Job drawing, mm, ordinate dimensions from the low corner. One solid piece. A direction names the side the tool comes from. Coordinates: 2 decimals unless noted, no trailing zeros. Loops run counter-clockwise (first coordinate to the right, second up) from the corner with the lowest first, then second, coordinate; pieces in that order, holes last. Notation, with made-up numbers: (57, 5.25) -> (63, 5.25) arc R26 cw to (63, 19.25) -> close; hole circle Ø5 at (75.5, 17.5). An arc over 180 degrees is marked (long way). Answer as CSV lines item,"result". Start each with the question number.
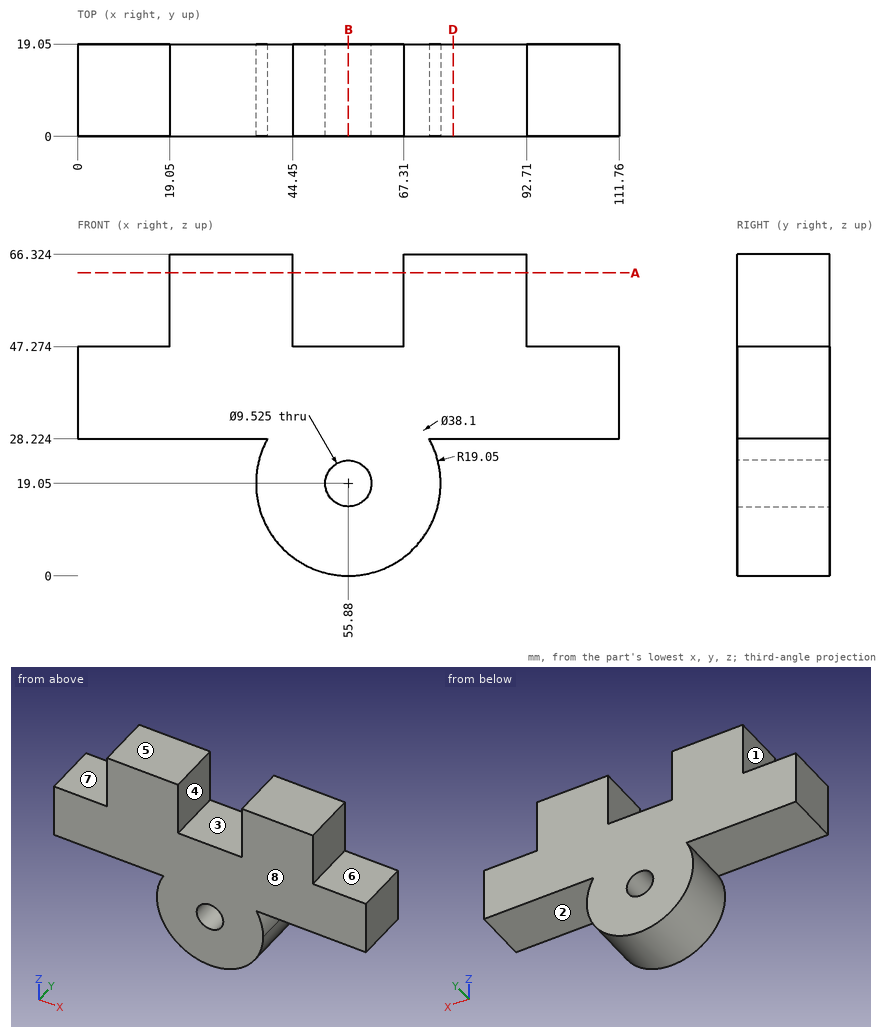
Q1. Two-plate mould, pull along X, no slides. Class the marked faces 1, 2 and 3: pulls with the +X half, pulls with the -X half, needs draft (parallel to the pull), parting line crosses it, or undercut.
Q2. Probe probe 1 along Z at (x, y) = (55.88, 5.5); probe 2 along Z at (x, y) = (95, 5.5); probe 3 along Z at (x, y) = (24.5, 14). List the from-to ranges inside material, lowest first. Write a range as from..to.
Q3. Which spindle directions (+Z, -Z, +X, -X, +Y, -Y) get a long thin tool onto all of the face, cutting with end or side? Do the marked faces 4, 5, 6, 7 and 8. Say none if no direction does.
Q4. Saw through at A-A (z = 62.5). List the corners of the cut face in (x, y), and give its area (3 significant figures).
Q5. Saw through at B-B (x = 55.88). List the corners of the cut face in (y, z).
Q6. Saw through at D-D (x = 77.5). List the corners of the cut face in (y, z).
Q7. Pin check, flat tips, straight feed: pin 1 Ø5.5 at (x, y) = (8, 7.5) entering from +Z; pin 2 Ø8 at (y, z) = (15.5, 23) entering from -X; pin 3 Ø2 at (y, z) = (2.5, 24) entering from +X. Stop position of each tip, or through.
Ans:
1,face 1,"pulls with the -X half"
1,face 2,"needs draft"
1,face 3,"undercut"
2,probe 1,"z = 0..14.29, 23.81..47.27"
2,probe 2,"z = 28.22..47.27"
2,probe 3,"z = 28.22..66.32"
3,face 4,"+Z, +Y, -Y"
3,face 5,"+Z, +X, -X, +Y, -Y"
3,face 6,"+Z, +X, +Y, -Y"
3,face 7,"+Z, -X, +Y, -Y"
3,face 8,"+Z, -Z, +X, -X, -Y"
4,outline,"(19.05, 0) -> (44.45, 0) -> (44.45, 19.05) -> (19.05, 19.05) -> close; (67.31, 0) -> (92.71, 0) -> (92.71, 19.05) -> (67.31, 19.05) -> close"
4,area,"968 mm²"
5,outline,"(0, 0) -> (19.05, 0) -> (19.05, 14.29) -> (0, 14.29) -> close; (0, 23.81) -> (19.05, 23.81) -> (19.05, 47.27) -> (0, 47.27) -> close"
6,outline,"(0, 28.22) -> (19.05, 28.22) -> (19.05, 66.32) -> (0, 66.32) -> close"
7,pin 1,"stops at z = 47.27"
7,pin 2,"stops at x = 36.83"
7,pin 3,"stops at x = 74.52"
